from build123d import *

# Parameters (mm, degrees)
SKETCH_1_R      = 5
EXTRUDE_1_DEPTH = 20
SKETCH_2_R      = 12.5
EXTRUDE_2_DEPTH = 5
EXTRUDE_START   = 10
SKETCH_3_R      = 12.5
SKETCH_3_R_2    = 9.15
EXTRUDE_3_DEPTH = 10
FILLET_1_R      = 5


with BuildPart() as part:
    # 草图1 → 凸台-拉伸1 (new body)
    with BuildSketch(Plane.XY):
        Circle(SKETCH_1_R)
    extrude(amount=EXTRUDE_1_DEPTH)

    # 草图2 → 凸台-拉伸2 (add)
    with BuildSketch(Plane(origin=(0, 0, 0), x_dir=(-1, 0, 0), z_dir=(0, 0, -1))):
        Circle(SKETCH_2_R)
    extrude(amount=EXTRUDE_2_DEPTH)

    # 草图3 → 凸台-拉伸3 (add)
    with BuildSketch(Plane.XY.offset(EXTRUDE_START)):
        Circle(SKETCH_3_R)
        Circle(SKETCH_3_R_2, mode=Mode.SUBTRACT)
    extrude(amount=-EXTRUDE_3_DEPTH)

    # 圆角1
    fillet_1_edges = [part.edges().sort_by_distance(p)[0] for p in [
        (12.5, 0, -5),
    ]]
    fillet(fillet_1_edges, radius=FILLET_1_R - 0.0001)  # a hair under: the kernel refuses the full size


solid = part.part
Build history of the part. All positions in model axes, mm. A direction names the side the tool comes from. Round coordinates to 2 decimals unless told otherwise and drop trailing zeros. Loops run counter-clockwise (first coordinate to the right, second up) from the corner with the lowest first, then second, coordinate; pieces in that order, holes last. Notation, with made-up numbers: (59.25, 59.5) -> (69.25, 59.5) arc R27 ccw to (69.25, 89.5) -> close; hole circle Ø6 at (-5.75, 32.5). An arc over 180 degrees is marked (long way). Use CSV: the item, a comma, the result in double quotes. Start each with the question number.
Q1. Which spindle directions (+Z, -Z, +X, -X, +Y, -Y) get a long thin tool onto all of the face, cutting with end or side? Do faces 3 (the face through (0, 0, -5)), 4 (the face through (-7, 7, 10)). Say none if no direction does.
Q2. Mould opens along Y. For faces 1 (the face through (0, 0, 20)), 2 (the face through (-1.08, -4.88, 9.86)) say: +Y half, -Y half, draft (parallel to the pull), parting line (faces both ways), or undercut.
Q3. Drill centre lines: L1, parallel to Y at x = 0, z = 4.75; L2, parallel to Y at x = 1, z = 8.75; L3, parallel to Z at x = 4.5, y = 2.25. Where is each one in solid material? Low to high.
Q4. Flat gauge pins, fed straight in: pin 1 Ø2 at (y, z) = (0.5, 10.5) entering from -X; pin 2 Ø12 at (y, z) = (8, 10) entering from -X; pin 3 Ø4 at (y, z) = (-3.5, 14) entering from -X; pin 4 Ø5 at (x, y) = (1, 9.5) entering from +Z. Where does each tip first touch, or does it go through?
Q5. Saw through at A-A on x = 0. Give the cut face in (y, z).
Q6. Saw through at B-B on z = 4. Give the cut face in (x, y).
Solutions:
1,face 3,"-Z, +X, -X, +Y, -Y"
1,face 4,"+Z"
2,face 1,"draft"
2,face 2,"undercut"
3,L1,"y = -12.5 to -9.15, -5 to 5, 9.15 to 12.5"
3,L2,"y = -12.46 to -9.1, -4.9 to 4.9, 9.1 to 12.46"
3,L3,"z = -5 to 0"
4,pin 1,"stops at x = -12.5"
4,pin 2,"stops at x = -12.34"
4,pin 3,"stops at x = -4.77"
4,pin 4,"stops at z = 10"
5,outline,"(-12.5, 0) arc R5 ccw to (-7.5, -5) -> (7.5, -5) arc R5 ccw to (12.5, 0) -> (12.5, 10) -> (9.15, 10) -> (9.15, 0) -> (5, 0) -> (5, 20) -> (-5, 20) -> (-5, 0) -> (-9.15, 0) -> (-9.15, 10) -> (-12.5, 10) -> close"
6,outline,"circle Ø25 at (0, 0); circle Ø10 at (0, 0); hole circle Ø18.3 at (0, 0)"
